```python
from build123d import *

# Parameters (mm, degrees)
SKETCH1_R           = 93.7895
SKETCH1_R_2         = 80.01
BOSS_EXTRUDE1_DEPTH = 6.35
SKETCH3_R           = 85.725
SKETCH3_R_2         = 80.01
BOSS_EXTRUDE2_DEPTH = 12.7


with BuildPart() as part:
    # Sketch1 → Boss-Extrude1 (new body, symmetric)
    with BuildSketch(Plane(origin=(0, 0, 0), x_dir=(1, 0, 0), z_dir=(0, 1, 0))):
        Circle(SKETCH1_R)
        Circle(SKETCH1_R_2, mode=Mode.SUBTRACT)
    extrude(amount=BOSS_EXTRUDE1_DEPTH, both=True)

    # Sketch3 → Boss-Extrude2 (add)
    with BuildSketch(Plane(origin=(0, 6.35, 0), x_dir=(1, 0, 0), z_dir=(0, 1, 0))):
        Circle(SKETCH3_R)
        Circle(SKETCH3_R_2, mode=Mode.SUBTRACT)
    boss_extrude2 = extrude(amount=BOSS_EXTRUDE2_DEPTH)

    # Mirror2: Boss-Extrude2 across plane
    add(boss_extrude2.mirror(Plane.ZX))


solid = part.part
```
The model under review builds one solid part; all positions refer to its coordinate system, in mm. A direction names the side the tool comes from. Give positions to 0.01 mm unless a question says otherwise; leave off trailing zeros. Loops run counter-clockwise (first coordinate to the right, second up) from the corner with the lowest first, then second, coordinate; pieces in that order, holes last. Notation, with made-up numbers: (25.5, -17) - (47.5, -17) arc R10 ccw to (47.5, -11) - close; hole circle Ø11 at (52, 37). An arc over 180 degrees is marked (long way). Answer as a JSON object with one key per item and string values.
Q1. Mouldability with a two-part tool opening along X and no side actions: class faces 1 (the cylindrical face through (76.315, 0.267, -24.033)), 2 (the flat face through (41, 6.35, 76)), 3 (the cylindrical face through (46.09, -12.61, -72.28)) as +X half, -X half, draft (parallel to the pull), parting line (faces both ways), or undercut.
Worked out:
{"face 1": "undercut", "face 2": "draft", "face 3": "parting line"}
Q2. Add section B-B on x = 62. State the section outline as (y, z) points, plus the area to 3 significant figures.
Worked out:
{"outline": "(-19.05, -59.2) - (-6.35, -59.2) - (-6.35, -70.37) - (6.35, -70.37) - (6.35, -59.2) - (19.05, -59.2) - (19.05, -50.57) - (-19.05, -50.57) - close; (-19.05, 50.57) - (19.05, 50.57) - (19.05, 59.2) - (6.35, 59.2) - (6.35, 70.37) - (-6.35, 70.37) - (-6.35, 59.2) - (-19.05, 59.2) - close", "area": "941 mm^2"}
Q3. Add section C-C on y = -13.5. State the section outline as (x, z) points (3 decimals).
Worked out:
{"outline": "circle Ø171.45 at (0, 0); hole circle Ø160.02 at (0, 0)"}
Q4. Insertion check: pin 1 (6 mm diameter, centred on x = -50, y = -15, fed in from -Z); pin 2 (12 mm diameter, centred on y = 0.5, z = 41, fed in from +X); pin 3 (1.5 mm diameter, centred on y = -2, z = -18, fed in from -X). Each pin has a flat end and moves straight along its axis. Give the tip position at first contact, or say it passes through.
Worked out:
{"pin 1": "stops at z = -71.69", "pin 2": "stops at x = 87.01", "pin 3": "stops at x = -92.19"}
Q5. For faces 4 (the cylindrical face through (89.46, 0.09, -28.17)), 5 (the cylindrical face through (46.09, 12.61, -72.28)), 6 (the flat face through (41, -6.35, 76)), list the 3-axis set-ups (+Z, -Z, +X, -X, +Y, -Y) from which the entire face can be reached by the end or side of a thin tool; tool diameter is ignored.
Worked out:
{"face 4": "+Y, -Y", "face 5": "+Y", "face 6": "-Y"}
Q6. Add section D-D on y = -3. State the section outline as (x, z) points.
Worked out:
{"outline": "circle Ø187.58 at (0, 0); hole circle Ø160.02 at (0, 0)"}
Q7. To check wall thickness, follow line 1 along Z through (x, y) = (2.5, 15); line 2 along X through (y, z) = (3, 0). State the ranges of each line that lie inside material, in increasing order.
Worked out:
{"line 1": "z = -85.69 to -79.97, 79.97 to 85.69", "line 2": "x = -93.79 to -80.01, 80.01 to 93.79"}
